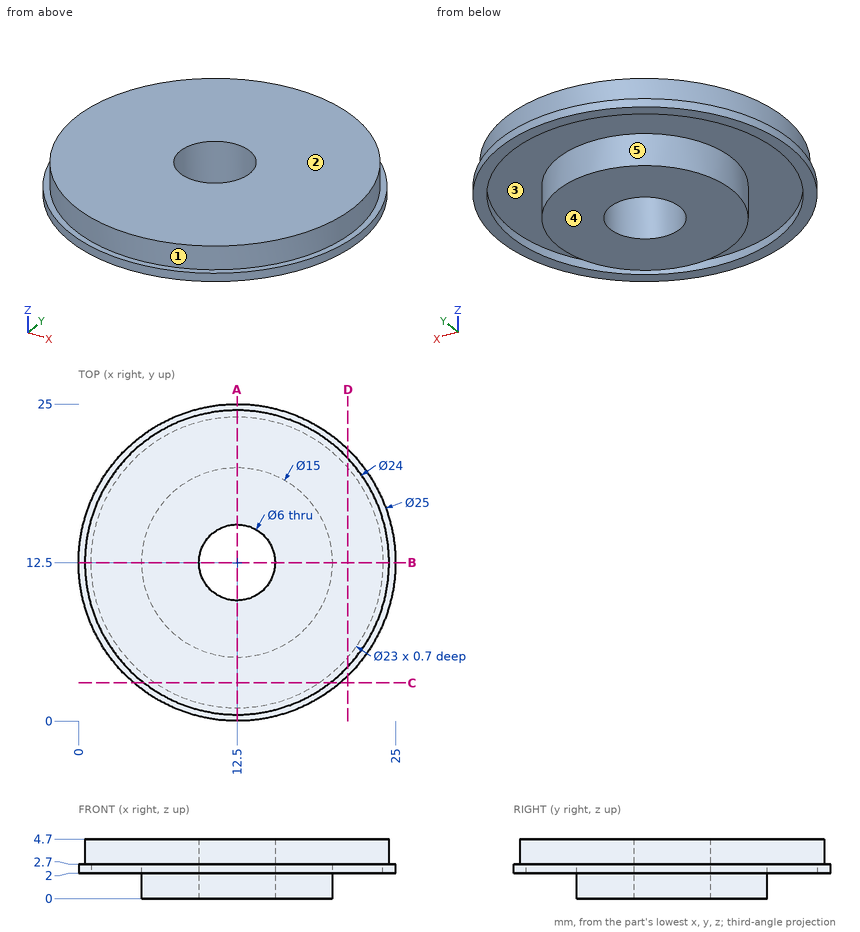
Geometry check sheet. Reference: drawing and pictorial views, mm from the part's lowest x, y, z. A direction names the side the tool comes from. Coordinates: 2 decimals unless noted, no trailing zeros. Order: outer loops, then holes, each group sorted by start corner. A loop starts at its lowest first (then second) coordinate and runs counter-clockwise, first axis right, second up.
Item 1: Scan lines: line 1 along Y through (x, z) = (12.5, 2.4); line 2 along Y through (x, z) = (12.5, 2.95); line 3 along Y through (x, z) = (9.75, 2.75). Record each from-to range of solid material in increasing order.
Item 2: Section check C-C (y = 3). Enter the section's corners in (x, z).
Item 3: Section check D-D (x = 21.25). Enter the section's corners in (y, z), plus the area to 3 significant figures.
Item 4: Mould release check, pull along Y, two halves, no side actions. Record for the marked faces 1, 2 and 3: released by +Y, released by -Y, zero draft, split by the parting line, or undercut.
Item 5: Depth check by flat-ended pin: pin 1 (1 mm diameter, centred on y = 17.5, z = 2.5, fed in from -X); pin 2 (1.5 mm diameter, centred on x = 6, z = 2.5, fed in from -Y); pin 3 (2 mm diameter, centred on y = 22.5, z = 4, fed in from -X). Enter the tip coordinate at first touch or a pass-through.
Item 6: Section check A-A (x = 12.5). Enter the section's corners in (y, z).
Item 7: Tool access check on the marked faces 4 and 5. Record the directions out of +Z, -Z, +X, -X, +Y, -Y that give a thin tool (end or side, any length) a straight path to the whole face; none if there is none.
Check sheet entries:
1. line 1: y = 0 to 1, 5 to 9.5, 15.5 to 20, 24 to 25
1. line 2: y = 0.5 to 9.5, 15.5 to 24.5
1. line 3: y = 0.82 to 11.3, 13.7 to 24.18
2. outline: (4.38, 2) - (6.02, 2) - (6.02, 2.7) - (18.98, 2.7) - (18.98, 2) - (20.62, 2) - (20.62, 2.7) - (19.83, 2.7) - (19.83, 4.7) - (5.17, 4.7) - (5.17, 2.7) - (4.38, 2.7) - close
3. outline: (3.57, 2) - (5.04, 2) - (5.04, 2.7) - (19.96, 2.7) - (19.96, 2) - (21.43, 2) - (21.43, 2.7) - (20.71, 2.7) - (20.71, 4.7) - (4.29, 4.7) - (4.29, 2.7) - (3.57, 2.7) - close
3. area: 34.9 mm2
4. face 1: split by the parting line
4. face 2: zero draft
4. face 3: undercut
5. pin 1: stops at x = 0.84
5. pin 2: stops at y = 1.4
5. pin 3: stops at x = 4.56
6. outline: (0, 2) - (1, 2) - (1, 2.7) - (5, 2.7) - (5, 0) - (9.5, 0) - (9.5, 4.7) - (0.5, 4.7) - (0.5, 2.7) - (0, 2.7) - close; (15.5, 0) - (20, 0) - (20, 2.7) - (24, 2.7) - (24, 2) - (25, 2) - (25, 2.7) - (24.5, 2.7) - (24.5, 4.7) - (15.5, 4.7) - close
7. face 4: -Z, +X, -X, +Y, -Y
7. face 5: -Z
